Job drawing, mm, ordinate dimensions from the low corner. One solid piece. Round coordinates to 2 decimals unless told otherwise and drop trailing zeros. Loops run counter-clockwise (first coordinate to the right, second up) from the corner with the lowest first, then second, coordinate; pieces in that order, holes last.
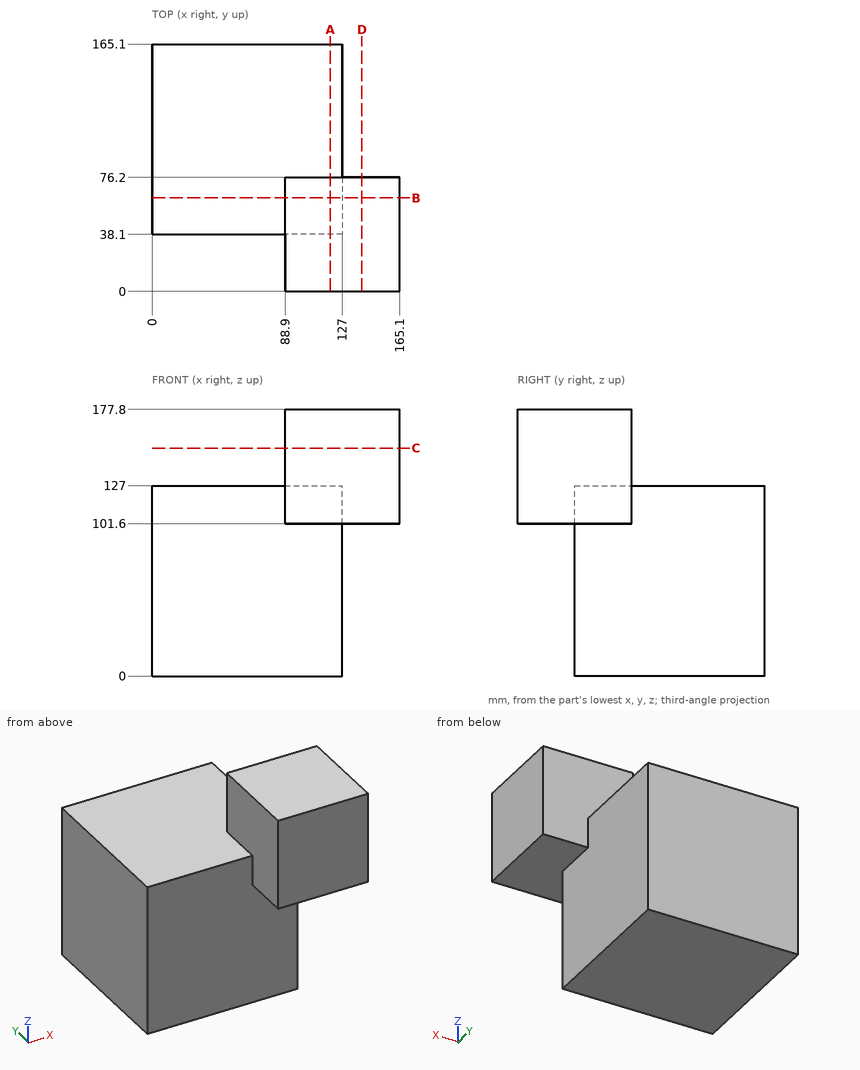
(1) Slice it at C-C on z = 152. List the corners of the cut face in (x, y).
Responses:
outline: (88.9, 0) - (165.1, 0) - (165.1, 76.2) - (88.9, 76.2) - close
(2) Slice it at D-D on x = 140. List the corners of the cut face in (y, z).
Responses:
outline: (0, 101.6) - (76.2, 101.6) - (76.2, 177.8) - (0, 177.8) - close
(3) Probe line 1 (X direction, y = 115, z = 108); line 2 (Y direction, x = 133, z = 156.5). List the from-to ranges inside material, lowest first.
Responses:
line 1: x = 0 to 127
line 2: y = 0 to 76.2
(4) Slice it at A-A on x = 119. List the corners of the cut face in (y, z), plus the area to 3 significant figures.
Responses:
outline: (0, 101.6) - (38.1, 101.6) - (38.1, 0) - (165.1, 0) - (165.1, 127) - (76.2, 127) - (76.2, 177.8) - (0, 177.8) - close
area: 21,000 mm2
(5) Slice it at B-B on y = 62.5. List the corners of the cut face in (x, z), plus the area to 3 significant figures.
Responses:
outline: (0, 0) - (127, 0) - (127, 101.6) - (165.1, 101.6) - (165.1, 177.8) - (88.9, 177.8) - (88.9, 127) - (0, 127) - close
area: 21,000 mm2
(6) Pin check, flat tip, straight feed: P1, Ø1, axis at x = 89, y = 130, coming from the +Z side. Stop position of the tip, or through.
Responses:
P1: stops at z = 127
